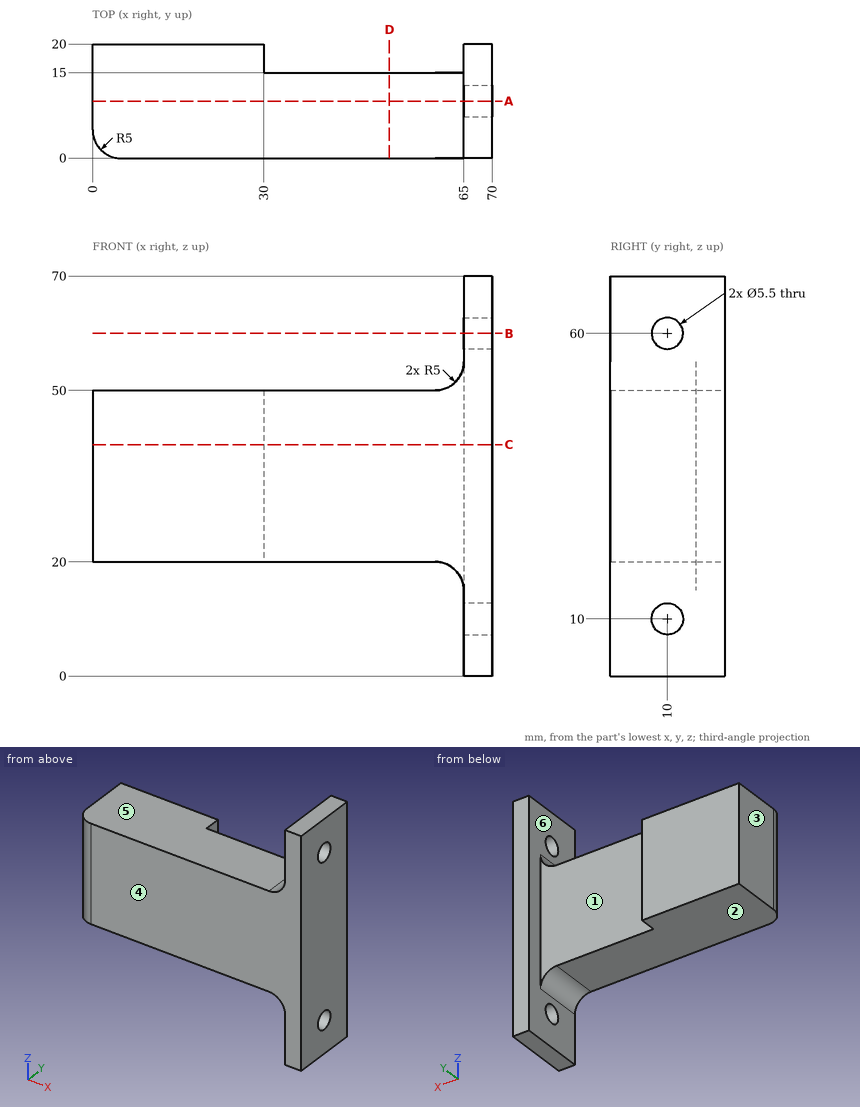
The drawing under review shows one solid part. Ordinate dimensions are in mm from its lowest x, y, z. A direction names the side the tool comes from. Coordinates: 2 decimals unless noted, no trailing zeros. Write each loop counter-clockwise with the first axis right and the second up, starting at its lowest first coordinate (ties: lowest second). Pieces come first, ordered by that corner, then holes. Notation, with made-up numbers: (-25.75, 31) - (-0.75, 31) arc R15 cw to (-0.75, 50) - close; hole circle Ø4 at (36, -20.5). An arc over 180 degrees is marked (long way). Put each result on its own line as item: value.
1. Add section C-C, the plane z = 40.5. Give the boundary of the cut face in (x, y), then the cut area to 3 significant figures.
Values found:
outline: (0, 5) arc R5 ccw to (5, 0) - (70, 0) - (70, 20) - (65, 20) - (65, 15) - (30, 15) - (30, 20) - (0, 20) - close
area: 1,220 mm²
2. Mouldability with a two-part tool opening along X and no side actions: class the marked faces 1, 2 and 3 as released by +X, released by -X, zero draft, split by the parting line, or undercut.
Values found:
face 1: undercut
face 2: zero draft
face 3: released by -X
3. Wall thickness on probe 1 along Y at (x, z) = (66.35, 60); probe 2 along X at (y, z) = (12.5, 65); probe 3 along Z at (x, y) = (30, 2.25): over which ranges is each line inside the solid? List them lowest first.
Values found:
probe 1: 0 to 7.25, 12.75 to 20
probe 2: 65 to 70
probe 3: 20 to 50
4. Machinability: for the marked faces 4, 5 and 6, which of the approach directions +Z, -Z, +X, -X, +Y, -Y give a long, thin tool a straight path to every point of the face, cutting with its end or side? Answer none if there is none.
Values found:
face 4: +Z, -Z, +X, -X, -Y
face 5: +Z, -X, +Y, -Y
face 6: +Y
5. Add section B-B, the plane z = 60. Give the boundary of the cut face in (x, y).
Values found:
outline: (65, 0) - (70, 0) - (70, 7.25) - (65, 7.25) - close; (65, 12.75) - (70, 12.75) - (70, 20) - (65, 20) - close
6. Add section A-A, the plane y = 10. Give the boundary of the cut face in (x, z), then the cut area to 3 significant figures.
Values found:
outline: (0, 20) - (60, 20) arc R5 cw to (65, 15) - (65, 12.75) - (70, 12.75) - (70, 57.25) - (65, 57.25) - (65, 55) arc R5 cw to (60, 50) - (0, 50) - close; (65, 0) - (70, 0) - (70, 7.25) - (65, 7.25) - close; (65, 62.75) - (70, 62.75) - (70, 70) - (65, 70) - close
area: 2,260 mm²
7. For pin 1 (3 mm diameter, centred on y = 7.5, z = 56.5, fed in from -X); pin 2 (12 mm diameter, centred on x = 8.5, z = 59.5, fed in from +Y) (3 decimals); pin 3 (6 mm diameter, centred on x = 14.5, y = 18, fed in from +Z); pin 4 (2 mm diameter, centred on x = 37.5, y = 12.5, fed in from -Z), all flat-tipped, find the tip position at first contact; note any pin that passes through.
Values found:
pin 1: x = 65
pin 2: through
pin 3: z = 50
pin 4: z = 20
8. Add section D-D, the plane x = 52. Give the boundary of the cut face in (y, z), then the cut area to 3 significant figures.
Values found:
outline: (0, 20) - (15, 20) - (15, 50) - (0, 50) - close
area: 450 mm²
